The listing builds one solid part. Answer for the finished solid, in the listing's coordinates (mm). A direction names the side the tool comes from. Round coordinates to 2 decimals unless told otherwise and drop trailing zeros. Loops run counter-clockwise (first coordinate to the right, second up) from the corner with the lowest first, then second, coordinate; pieces in that order, holes last. Notation, with made-up numbers: (33, -22.75) - (62, -22.75) arc R16 cw to (62, -0.75) - close; hole circle Ø8 at (78.25, 65.25). An arc over 180 degrees is marked (long way). One line per item, written item: value.
```python
from build123d import *

# Parameters (mm, degrees)
ESQUISSE1_W             = 190
ESQUISSE1_H             = 220
ESQUISSE1_R             = 65
BOSS_EXTRU_1_DEPTH      = 31
ESQUISSE2_R             = 5
ENL_V_MAT_EXTRU_1_DEPTH = 15
ESQUISSE4_W             = 150
ESQUISSE4_H             = 150
ESQUISSE4_R             = 55
BOSS_EXTRU_2_DEPTH      = 10
CONG_1_R                = 2


with BuildPart() as part:
    # Esquisse1 → Boss.-Extru.1 (new body)
    with BuildSketch(Plane.XY):
        with Locations((0, 110)):
            Rectangle(ESQUISSE1_W, ESQUISSE1_H)
        with Locations((0, 95)):
            Circle(ESQUISSE1_R, mode=Mode.SUBTRACT)
    extrude(amount=BOSS_EXTRU_1_DEPTH)

    # Esquisse2 → Enlèv. mat.-Extru.1 (cut)
    with BuildSketch(Plane(origin=(0, 220, 0), x_dir=(1, 0, 0), z_dir=(0, 1, 0))):
        with Locations(Location((-80, -15.5, 0), (0, 0, 180))):
            Circle(ESQUISSE2_R)
    enl_v_mat_extru_1 = extrude(amount=-ENL_V_MAT_EXTRU_1_DEPTH, mode=Mode.SUBTRACT)

    # Symétrie1: Enlèv. mat.-Extru.1 across plane
    add(enl_v_mat_extru_1.mirror(Plane(origin=(0, 0, 0), x_dir=(0, 0, 1), z_dir=(1, 0, 0))), mode=Mode.SUBTRACT)

    # Esquisse4 → Boss.-Extru.2 (add)
    with BuildSketch(Plane.XY):
        with Locations((0, 95)):
            Rectangle(ESQUISSE4_W, ESQUISSE4_H)
        with Locations((0, 95)):
            Circle(ESQUISSE4_R, mode=Mode.SUBTRACT)
    extrude(amount=-BOSS_EXTRU_2_DEPTH)

    # Congé1
    cong_1_edges = [part.edges().sort_by_distance(p)[0] for p in [
        (-55, 95, -10),
        (75, 95, 0),
        (0, 170, 0),
        (-75, 95, 0),
        (0, 20, 0),
    ]]
    fillet(cong_1_edges, radius=CONG_1_R)


solid = part.part
```
1) For a pull along Y with two mould halves and no side action, classify faces 5 (the flat face through (-80, 205, 16)), 6 (the cylindrical face through (-11.923, 41.308, -3.944)), 7 (the flat face through (-1, 20, -6)), 8 (the cylindrical face through (-84.619, 212.605, 13.585)) as released by +Y, released by -Y, zero draft, split by the parting line, or undercut.
Final values:
face 5: released by +Y
face 6: undercut
face 7: released by -Y
face 8: zero draft
2) Consider L1, parallel to Y at x = -0.5, z = 26.5; L2, parallel to Z at x = 80, y = 211.5; L3, parallel to Z at x = -79, y = 120.5. Determine where each line is inside the solid, lowest interval first.
Final values:
L1: 0 to 30, 160 to 220
L2: 0 to 10.5, 20.5 to 31
L3: 0 to 31
3) Each of these flat-tipped pins is pushed along its axis until it touches: pin 1 Ø4 at (x, z) = (-21, -2.5) entering from +Y; pin 2 Ø11 at (x, z) = (80.5, 14.5) entering from +Y; pin 3 Ø2.5 at (y, z) = (79, -7) entering from +X; pin 4 Ø1.5 at (x, y) = (-58.5, 90.5) entering from +Z. Where does it stop, or does it pass through?
Final values:
pin 1: y = 170.68
pin 2: y = 220
pin 3: x = 75
pin 4: z = 0
4) A cutting plane is placed at B-B on y = 95. Give the vertices of the cut face in (x, z), and give its area (3 significant figures).
Final values:
outline: (-95, 0) - (-77, 0) arc R2 cw to (-75, -2) - (-75, -10) - (-57, -10) arc R2 ccw to (-55, -8) - (-55, 0) - (-65, 0) - (-65, 31) - (-95, 31) - close; (55, -8) arc R2 ccw to (57, -10) - (75, -10) - (75, -2) arc R2 cw to (77, 0) - (95, 0) - (95, 31) - (65, 31) - (65, 0) - (55, 0) - close
area: 2,260 mm2
5) For faces 1 (the flat face through (-1, 170, -6)), 2 (the flat face through (-1, 185, 0)), 3 (the flat face through (75, 94, -6)), 4 (the cylindrical face through (84.619, 212.605, 13.585)), determine the directions among +Z, -Z, +X, -X, +Y, -Y from which every point of the face is accessible in a straight line to the end or side of a thin tool.
Final values:
face 1: -Z, +X, -X, +Y
face 2: -Z
face 3: -Z, +X, +Y, -Y
face 4: +Y
6) A cutting plane is placed at A-A on x = 0. Give the vertices of the cut face in (y, z).
Final values:
outline: (0, 0) - (18, 0) arc R2 cw to (20, -2) - (20, -10) - (38, -10) arc R2 ccw to (40, -8) - (40, 0) - (30, 0) - (30, 31) - (0, 31) - close; (150, -8) arc R2 ccw to (152, -10) - (170, -10) - (170, -2) arc R2 cw to (172, 0) - (220, 0) - (220, 31) - (160, 31) - (160, 0) - (150, 0) - close
7) A cutting plane is placed at D-D on y = 25. Give the vertices of the cut face in (x, z), and give its area (3 significant figures).
Final values:
outline: (-95, 0) - (-77, 0) arc R2 cw to (-75, -2) - (-75, -10) - (75, -10) - (75, -2) arc R2 cw to (77, 0) - (95, 0) - (95, 31) - (-95, 31) - close
area: 7,390 mm2
8) A cutting plane is placed at C-C on z = 15.5. Give the vertices of the cut face in (x, y), and give its area (3 significant figures).
Final values:
outline: (-95, 0) - (95, 0) - (95, 220) - (85, 220) - (85, 205) - (75, 205) - (75, 220) - (-75, 220) - (-75, 205) - (-85, 205) - (-85, 220) - (-95, 220) - close; hole circle Ø130 at (0, 95)
area: 28,200 mm2
